Read the model definition and answer for the solid it produces. Units are mm, in the model's axes. Face numbers are marked on the shaded views. Round coordinates to 2 decimals unless told otherwise and drop trailing zeros. Order: outer loops, then holes, each group sorted by start corner. A loop starts at its lowest first (then second) coordinate and runs counter-clockwise, first axis right, second up.
from build123d import *

# Parameters (mm, degrees)
PAD039_DEPTH           = 5
THICKNESS001_T         = -1.5
SKETCH099_R            = 1.5
POCKET045_DEPTH        = 5
SKETCH100_R            = 1.5
PAD040_DEPTH           = 3
LINEARPATTERN001_COUNT = 4
LINEARPATTERN001_PITCH = 50
SKETCH102_R            = 4
SKETCH102_R_2          = 2
PAD041_DEPTH           = 3.5


with BuildPart() as part:
    # Sketch098 → Pad039 (new body)
    with BuildSketch(Plane.XY):
        with BuildLine():
            Line((18.090053, -27), (229.701779, -27))
            ThreePointArc((229.701779, 27), (218, 0), (229.701779, -27))
            Line((229.701779, 27), (18.090053, 27))
            ThreePointArc((24.804234, 21), (21.655945, 24.233655), (18.090053, 27))
            Line((36.520259, 21), (24.804234, 21))
            ThreePointArc((36.520259, -21), (46, 0), (36.520259, 21))
            Line((36.520259, -21), (24.804234, -21))
            ThreePointArc((18.090053, -27), (21.655945, -24.233655), (24.804234, -21))
        make_face()
    extrude(amount=PAD039_DEPTH)

    # Thickness001
    thickness001_openings = [part.faces().sort_by_distance(p)[0] for p in [
        (129.781402, 0, 5),
    ]]
    offset(amount=THICKNESS001_T, openings=thickness001_openings)

    # Sketch099 (on Face9 of Pad039) → Pocket045 (cut)
    with BuildSketch(Plane(origin=(0, 0, 0), x_dir=(1, 0, 0), z_dir=(0, 0, -1))):
        with Locations((48, 22)):
            Circle(SKETCH099_R)
        with Locations((48, -22)):
            Circle(SKETCH099_R)
    pocket045 = extrude(amount=-POCKET045_DEPTH, mode=Mode.SUBTRACT)

    # Sketch100 (on Face23 of Pocket045) → Pad040 (join)
    with BuildSketch(Plane.XY.offset(1.5)):
        with BuildLine():
            ThreePointArc((45, 22), (48.000011, 19), (51, 22.000022))
            Line((51, 22.000022), (51, 25.5))
            Line((45, 25.5), (51, 25.5))
            Line((45, 25.5), (45, 22))
        make_face()
        with Locations((48, 22)):
            Circle(SKETCH100_R, mode=Mode.SUBTRACT)
        with BuildLine():
            ThreePointArc((51, -22), (48, -19), (45, -22))
            Line((45, -22), (45, -25.5))
            Line((45, -25.5), (51, -25.5))
            Line((51, -22), (51, -25.5))
        make_face()
        with Locations((48, -22)):
            Circle(SKETCH100_R, mode=Mode.SUBTRACT)
    pad040 = extrude(amount=PAD040_DEPTH)

    # LinearPattern001: Pocket045, Pad040 ×4
    with Locations(*[(i * LINEARPATTERN001_PITCH, 0, 0) for i in range(1, LINEARPATTERN001_COUNT)]):
        add(pocket045, mode=Mode.SUBTRACT)
        add(pad040)

    # Sketch102 (on Face25 of LinearPattern001) → Pad041 (join)
    with BuildSketch(Plane.XY.offset(1.5)):
        with Locations((66.39682, 15.867146)):
            Circle(SKETCH102_R)
        with Locations((66.39682, 15.867146)):
            Circle(SKETCH102_R_2, mode=Mode.SUBTRACT)
        with Locations((81.342545, -15.126509)):
            Circle(SKETCH102_R)
        with Locations((81.342545, -15.126509)):
            Circle(SKETCH102_R_2, mode=Mode.SUBTRACT)
    extrude(amount=PAD041_DEPTH)


with BuildPart() as part_1:
    # Body011 placement: moved
    add(part.part.moved(Location((5, 0, -20))))


solid = part_1.part
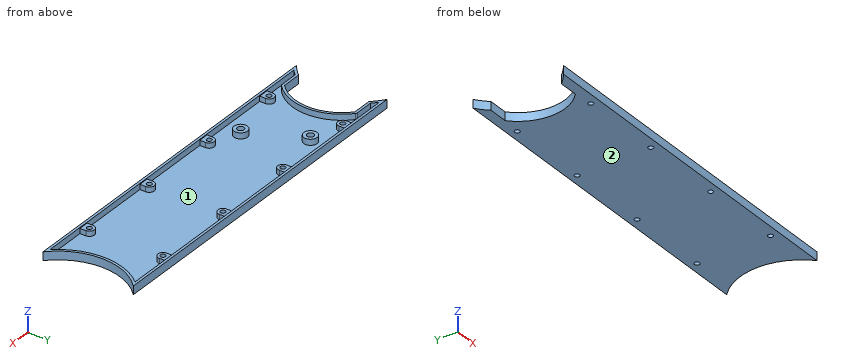
Q1. A cutting plane is placed at A-A, the plane x = 124.5. Give the vertices of the cut face in (y, z).
Outcome:
outline: (-27, -20) - (27, -20) - (27, -15) - (25.5, -15) - (25.5, -18.5) - (-25.5, -18.5) - (-25.5, -15) - (-27, -15) - close
Q2. A cutting plane is placed at B-B, the plane y = 4. Give the vertices of the cut face in (x, z), plus the area to 3 significant figures.
Outcome:
outline: (50.71, -20) - (223.22, -20) - (223.22, -15) - (221.71, -15) - (221.71, -18.5) - (52.23, -18.5) - (52.23, -15) - (50.71, -15) - close
area: 269 mm2
Q3. Flat-ended cylindrical pins translate along their axes: pin 1 (3 mm diameter, centred on y = -8, z = -19, fed in from +X); pin 2 (1.2 mm diameter, centred on x = 72, y = 16.5, fed in from +Z); pin 3 (5 mm diameter, centred on x = 204, y = 21.5, fed in from +Z); pin 4 (2.5 mm diameter, centred on x = 203, y = 22, fed in from -Z). Find the tip coordinate at first contact, or state that the pin passes through.
Outcome:
pin 1: stops at x = 224.24
pin 2: stops at z = -18.5
pin 3: stops at z = -15.5
pin 4: passes through
Q4. A cutting plane is placed at C-C, the plane z = -17.2. Give the number of separate pieces and of enclosed holes in the cut face, plus the area to 3 significant figures.
Outcome:
separate pieces: 3
enclosed holes: 11
area: 1,140 mm2
Q5. For a pull along X with two mould halves and no side action, classify the marked faces 1 and 2 as released by +X, released by -X, zero draft, split by the parting line, or undercut.
Outcome:
face 1: undercut
face 2: zero draft
Q6. Straight lines are drawn through the part: probe 1 along Y at (x, z) = (203, -16.95); probe 2 along Y at (x, z) = (66, -17.2); probe 3 along Y at (x, z) = (153, -18.6). For each, find the intervals that lie inside material, in ascending order.
Outcome:
probe 1: y = -27 to -23.5, -20.5 to -19, 19 to 20.5, 23.5 to 27
probe 2: y = -27 to -25.5, 25.5 to 27
probe 3: y = -27 to -23.5, -20.5 to 20.5, 23.5 to 27
